The figure shows three views and two pictorial views of one solid part (mm, origin at its lowest corner). Answer the questions. A direction names the side the tool comes from. Give positions to 0.01 mm unless a question says otherwise; leave off trailing zeros. Write each loop counter-clockwise with the first axis right and the second up, starting at its lowest first coordinate (ties: lowest second). Pieces come first, ordered by that corner, then holes. Notation, with made-up numbers: (48.5, -28.5) - (81.5, -28.5) arc R11 ccw to (81.5, -13.5) - close; hole circle Ø4 at (78.5, 33.5). An arc over 180 degrees is marked (long way). Use a Markdown table: item, result. Add a question column.
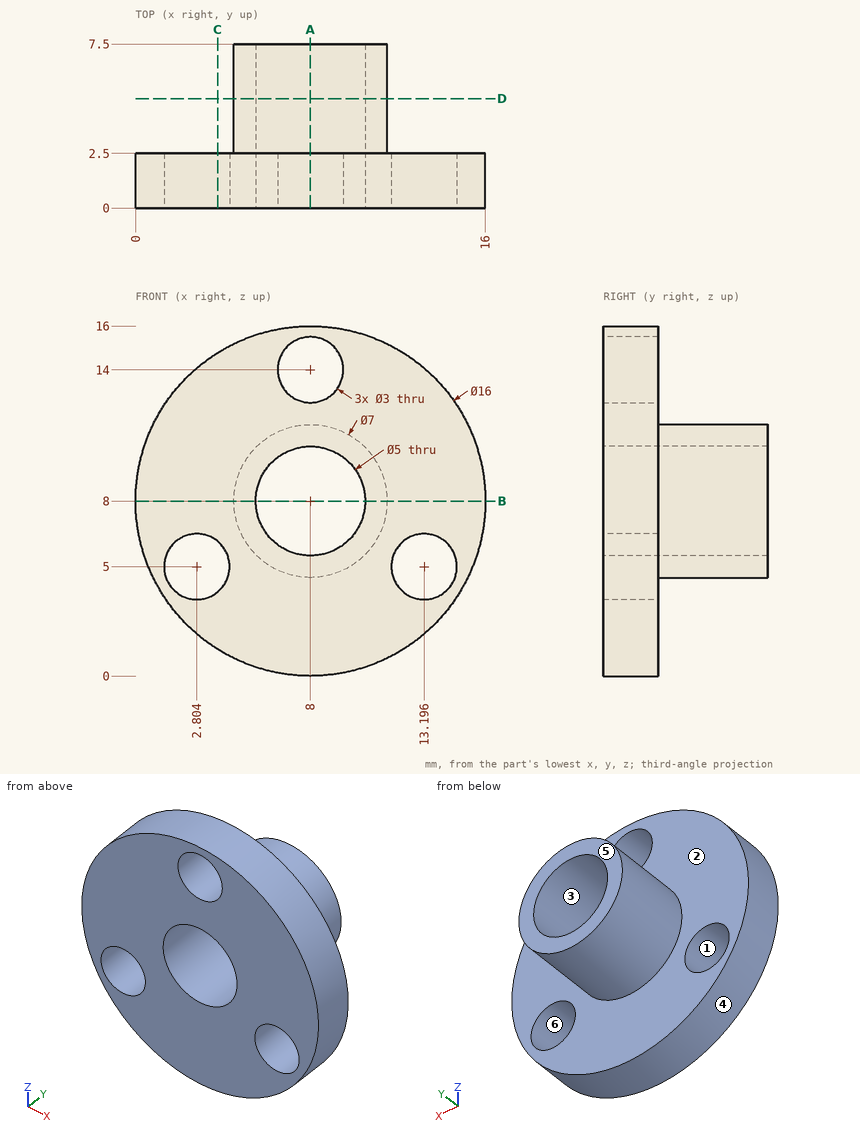
1. For a pull along Z with two mould halves and no side action, classify the marked faces 3, 4, 5 and 6 as released by +Z, released by -Z, zero draft, split by the parting line, or undercut.
2. Consider L1, parallel to X at y = 5.5, z = 8; L2, parallel to X at y = 1.2, z = 5; L3, parallel to X at y = 1.5, z = 8. Determine where each line is inside the solid, lowest interval first. Write a range as [from, to].
3. The part is cut by section A-A (x = 8). Give the vertices of the cut face in (y, z), and give its area (3 significant figures).
4. The part is cut by section B-B (z = 8). Give the vertices of the cut face in (x, y), and give its area (3 significant figures).
5. The part is cut by section D-D (y = 5). Give the vertices of the cut face in (x, z).
6. Which of the six approach directions +Z, -Z, +X, -X, +Y, -Y give full straight-line access (tool end or side, diameter ignored) to the marked faces 1 and 2?
7. The part is cut by section C-C (x = 3.75). Give the vertices of the cut face in (y, z), and give its area (3 significant figures).
8. Given P1, Ø2, axis at x = 13, y = 3, coming from the +Z side; P2, Ø1.5, axis at y = 5.5, z = 6.5, coming from the +X side; P3, Ø1, axis at x = 8.5, y = 4, coming from the -Z side, each flat-ended and moving along its own axis, determine where each tip first touches the part or whether it passes through.
Check values:
| question | item | result |
|---|---|---|
| 1 | face 3 | undercut |
| 1 | face 4 | split by the parting line |
| 1 | face 5 | zero draft |
| 1 | face 6 | undercut |
| 2 | L1 | x = [4.5, 5.5], [10.5, 11.5] |
| 2 | L2 | x = [0.58, 1.3], [4.3, 11.7], [14.7, 15.42] |
| 2 | L3 | x = [0, 5.5], [10.5, 16] |
| 3 | outline | (0, 0) - (2.5, 0) - (2.5, 4.5) - (7.5, 4.5) - (7.5, 5.5) - (0, 5.5) - close; (0, 10.5) - (7.5, 10.5) - (7.5, 11.5) - (2.5, 11.5) - (2.5, 12.5) - (0, 12.5) - close; (0, 15.5) - (2.5, 15.5) - (2.5, 16) - (0, 16) - close |
| 3 | area | 30.0 mm2 |
| 4 | outline | (0, 0) - (5.5, 0) - (5.5, 7.5) - (4.5, 7.5) - (4.5, 2.5) - (0, 2.5) - close; (10.5, 0) - (16, 0) - (16, 2.5) - (11.5, 2.5) - (11.5, 7.5) - (10.5, 7.5) - close |
| 4 | area | 37.5 mm2 |
| 5 | outline | circle Ø7 at (8, 8); hole circle Ø5 at (8, 8) |
| 6 | face 1 | +Y, -Y |
| 6 | face 2 | +Y |
| 7 | outline | (0, 1.22) - (2.5, 1.22) - (2.5, 3.84) - (0, 3.84) - close; (0, 6.16) - (2.5, 6.16) - (2.5, 14.78) - (0, 14.78) - close |
| 7 | area | 28.1 mm2 |
| 8 | P1 | stops at z = 14.85 |
| 8 | P2 | stops at x = 11.42 |
| 8 | P3 | stops at z = 4.5 |
